Geometry: see drawing. Coordinates: mm, zero at the bounding-box minimum. A direction names the side the tool comes from. Coordinates: 2 decimals unless noted, no trailing zeros. Loops run counter-clockwise (first coordinate to the right, second up) from the corner with the lowest first, then second, coordinate; pieces in that order, holes last. Notation, with made-up numbers: (21.25, -10.5) -> (39.25, -10.5) arc R17 cw to (39.25, 17.5) -> close; hole circle Ø9 at (-22, -14). An arc over 180 degrees is marked (long way). One line per question, with ' | ' between items. Start each with the question number.
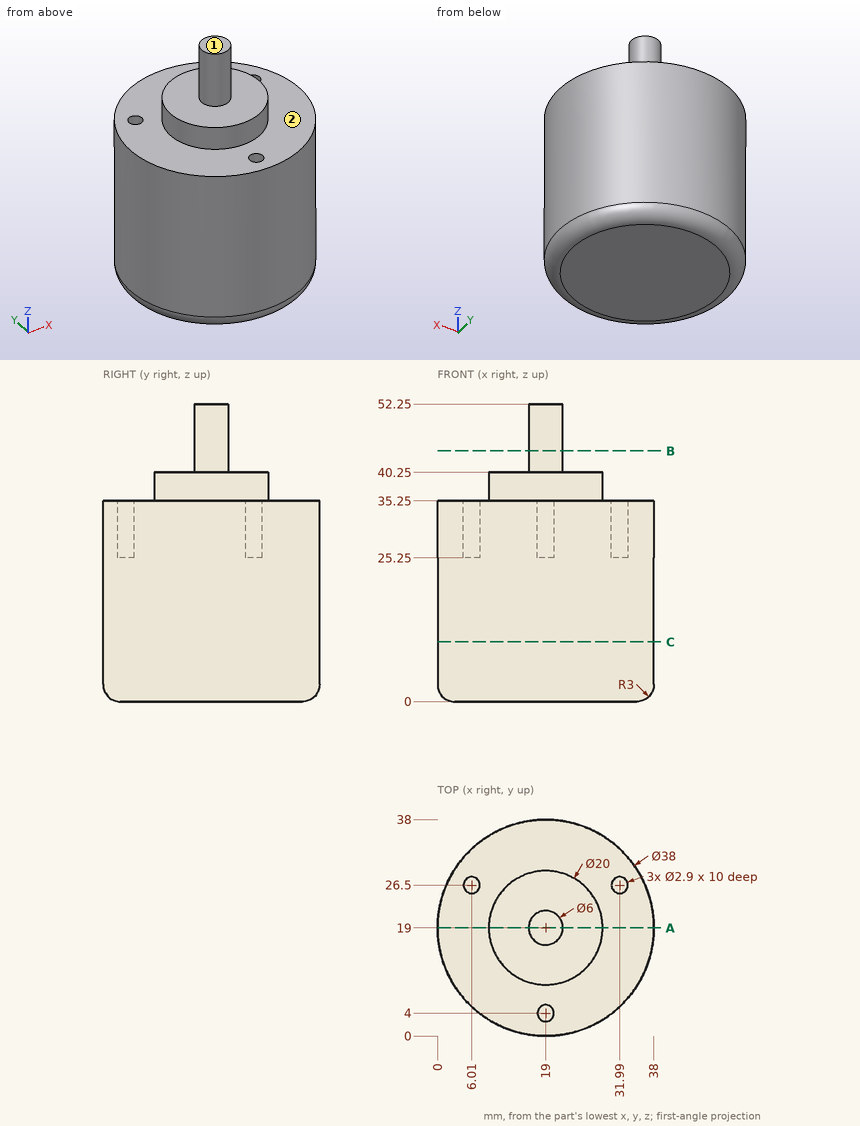
(1) Ray query, L1, parallel to X at y = 26, z = 28; L2, parallel to Z at x = 25.5, y = 7.5; L3, parallel to Y at x = 6.5, z = 30.5 (1 decimal). Return the intervals inside material, ascending.
(2) Cut plane C-C, the plane z = 10.5. Return the cut outline in (x, y).
(3) Contact query for flat-ended pins moving along their axis: pin 1 Ø10 at (x, z) = (6.5, 14) entering from -Y; pin 2 Ø5 at (x, z) = (5.5, 14) entering from -Y; pin 3 Ø4 at (x, y) = (6.01, 26.5) entering from -Z; pin 4 Ø3.5 at (x, y) = (19, 4) entering from +Z. Output: stop coordinate, or through.
(4) Cut plane B-B, the plane z = 44. Return the cut outline in (x, y), and give its area (3 significant figures).
(5) Access query for the marked faces 1 and 2. Directions: +Z, -Z, +X, -X, +Y, -Y. A direction counts if a zero-diameter tool reaches every point of the face in a straight line with its end or side. Return the directions, or none.
(6) Cut plane A-A, the plane y = 19. Return the cut outline in (x, z).
Here are the results:
1) L1: x = 1.34 to 4.65, 7.37 to 30.63, 33.35 to 36.66 | L2: z = 0 to 35.25 | L3: y = 4.7 to 25.1, 27.9 to 33.3
2) outline: circle Ø38 at (19, 19)
3) pin 1: stops at y = 1.54 | pin 2: stops at y = 3.51 | pin 3: stops at z = 0 | pin 4: stops at z = 35.25
4) outline: circle Ø6 at (19, 19) | area: 28.3 mm2
5) face 1: +Z, +X, -X, +Y, -Y | face 2: +Z
6) outline: (0, 3) arc R3 ccw to (3, 0) -> (35, 0) arc R3 ccw to (38, 3) -> (38, 35.25) -> (29, 35.25) -> (29, 40.25) -> (22, 40.25) -> (22, 52.25) -> (16, 52.25) -> (16, 40.25) -> (9, 40.25) -> (9, 35.25) -> (0, 35.25) -> close
